from build123d import *

# Parameters (mm, degrees)
EXTRUDE_1_DEPTH     = 1.5
CHAMFER_1_SIZE      = 4
SKETCH_2_R          = 1
CUT_EXTRUDE_1_DEPTH = 130.838515087
SKETCH_3_R          = 2.1
CUT_EXTRUDE_2_DEPTH = 130.838515087
CHAMFER_2_SIZE      = 2


with BuildPart() as part:
    # 草图1 → 凸台-拉伸1 (new, symmetric)
    with BuildSketch(Plane.XY):
        Polygon((-49, -120.2), (-29, -120.2), (-29, -14.8), (49, -14.8), (49, 120.2), (-49, 120.2), (-49, -14.8), align=None)
    extrude(amount=EXTRUDE_1_DEPTH, both=True)

    # 倒角1
    chamfer_1_edges = [part.edges().sort_by_distance(p)[0] for p in [
        (-49, 120.2, 0),
        (49, 120.2, 0),
        (49, -14.8, 0),
        (-29, -120.2, 0),
        (-49, -120.2, 0),
    ]]
    chamfer(chamfer_1_edges, length=CHAMFER_1_SIZE)

    # 草图2 → 切除-拉伸1 (cut, through all)
    with BuildSketch(Plane.XY.offset(1.5)):
        with Locations((-28, -14.8)):
            Circle(SKETCH_2_R)
    extrude(amount=-CUT_EXTRUDE_1_DEPTH, mode=Mode.SUBTRACT)

    # 草图3 → 切除-拉伸2 (cut, through all)
    with BuildSketch(Plane.XY.offset(1.5)):
        with Locations((-39, -110.2)):
            Circle(SKETCH_3_R)
        with Locations((-39, -24.8)):
            Circle(SKETCH_3_R)
    extrude(amount=-CUT_EXTRUDE_2_DEPTH, mode=Mode.SUBTRACT)

    # 倒角2
    chamfer_2_edges = [part.edges().sort_by_distance(p)[0] for p in [
        (-41.1, -110.2, -1.5),
        (-41.1, -24.8, -1.5),
    ]]
    chamfer(chamfer_2_edges, length=CHAMFER_2_SIZE)


solid = part.part
For this review, take the finished solid that the model builds, in its own axes (mm). Give positions to 0.01 mm unless a question says otherwise; leave off trailing zeros. Order: outer loops, then holes, each group sorted by start corner. A loop starts at its lowest first (then second) coordinate and runs counter-clockwise, first axis right, second up. Notation, with made-up numbers: (54, 78.25) - (104, 78.25) arc R33 ccw to (104, 116.25) - close; hole circle Ø8 at (-4.75, 42.25). An arc over 180 degrees is marked (long way). Answer as a JSON object with one key per item and string values. Group by question number.
Item 1: Take a section at A-A on x = -39. Give the boundary of the cut face in (y, z), and give its area (3 significant figures).
Item 2: Draft analysis for pull direction Y (two halves, no side actions). For faces 1 (the flat face through (-47, 118.2, 0)), 2 (the flat face through (-12, 28, -1.5)), 3 (the cylindrical face through (-39.273, -108.118, 1.007)), state which applies: pulls with the +Y half, pulls with the -Y half, needs draft (parallel to the pull), parting line crosses it, or undercut.
Item 3: Take a section at C-C on z = -0.7. Give the boundary of the cut face in (x, y).
Item 4: Clearance check with flat-ended pins moving along their axes: pin 1 Ø3.5 at (x, y) = (-39, -24.8) entering from +Z; pin 2 Ø1.5 at (x, z) = (21, -0.5) entering from -Y; pin 3 Ø0.9 at (y, z) = (-61, 0.5) entering from +X. State where each tip first meets the part, or that it passes through.
Item 5: Take a section at D-D on y = -52. Give the boundary of the cut face in (x, z), and give its area (3 significant figures).
Item 6: Wall thickness on line 1 along Y through (x, z) = (-39, 0.75); line 2 along Y through (x, z) = (13.5, 1.15); line 3 along X through (y, z) = (-24, 0.6): over which ranges is each line inside the solid? List them lowest first.
Item 7: Take a section at B-B on y = -24.8. Give the boundary of the cut face in (x, z).
Reported:
{
 "1": {"outline": "(-120.2, -1.5) - (-114.3, -1.5) - (-112.3, 0.5) - (-112.3, 1.5) - (-120.2, 1.5) - close; (-108.1, 0.5) - (-106.1, -1.5) - (-28.9, -1.5) - (-26.9, 0.5) - (-26.9, 1.5) - (-108.1, 1.5) - close; (-22.7, 0.5) - (-20.7, -1.5) - (120.2, -1.5) - (120.2, 1.5) - (-22.7, 1.5) - close", "area": "688 mm^2"},
 "2": {"face 1": "pulls with the +Y half", "face 2": "needs draft", "face 3": "undercut"},
 "3": {"outline": "(-49, -116.2) - (-45, -120.2) - (-33, -120.2) - (-29, -116.2) - (-29, -14.8) arc R1 cw to (-27, -14.8) - (45, -14.8) - (49, -10.8) - (49, 116.2) - (45, 120.2) - (-45, 120.2) - (-49, 116.2) - close; hole circle Ø6.6 at (-39, -110.2); hole circle Ø6.6 at (-39, -24.8)"},
 "4": {"pin 1": "through", "pin 2": "y = -14.8", "pin 3": "x = -29"},
 "5": {"outline": "(-49, -1.5) - (-29, -1.5) - (-29, 1.5) - (-49, 1.5) - close", "area": "60.0 mm^2"},
 "6": {"line 1": "-120.2 to -112.3, -108.1 to -26.9, -22.7 to 120.2", "line 2": "-14.8 to 120.2", "line 3": "-49 to -40.94, -37.06 to -29"},
 "7": {"outline": "(-49, -1.5) - (-43.1, -1.5) - (-41.1, 0.5) - (-41.1, 1.5) - (-49, 1.5) - close; (-36.9, 0.5) - (-34.9, -1.5) - (-29, -1.5) - (-29, 1.5) - (-36.9, 1.5) - close"}
}
